from build123d import *

# Parameters (mm, degrees)
ESQUISSE2_W    = 4
ESQUISSE2_H    = 2
ESQUISSE2_W_2  = 2
ESQUISSE2_H_2  = 4
ENCOCHES_DEPTH = 24.34523506


with BuildPart() as part:
    # Esquisse1 → Base (revolve)
    with BuildSketch(Plane.XY, mode=Mode.PRIVATE) as base_sk:
        Polygon((7.633974596, 5), (14, 5), (14, 1.154700538), (12, 0), (7.633974596, 0), align=None)
    revolve(base_sk.sketch.rotate(Axis((0, 0, 0), (0, 1, 0)), 90), axis=Axis((0, 0, 0), (0, 1, 0)))

    # Esquisse2 → Encoches (cut, through all)
    with BuildSketch(Plane(origin=(0, 5, -4), x_dir=(1, 0, 0), z_dir=(0, -1, 0))):
        with Locations((0, -9)):
            Rectangle(ESQUISSE2_W, ESQUISSE2_H)
        with Locations((0, 17)):
            Rectangle(ESQUISSE2_W, ESQUISSE2_H)
        with Locations((13, 4)):
            Rectangle(ESQUISSE2_W_2, ESQUISSE2_H_2)
        with Locations((-13, 4)):
            Rectangle(ESQUISSE2_W_2, ESQUISSE2_H_2)
    extrude(amount=ENCOCHES_DEPTH, mode=Mode.SUBTRACT)


solid = part.part
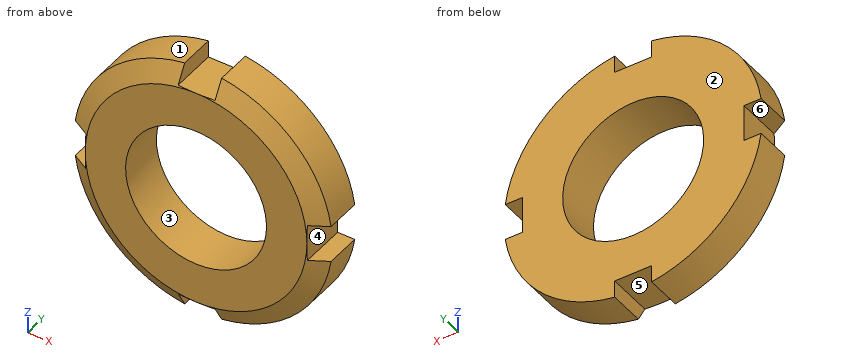
Build history of the part. All positions in model axes, mm. Face numbers are marked on the shaded views. A direction names the side the tool comes from. Coordinates: 2 decimals unless noted, no trailing zeros. Order: outer loops, then holes, each group sorted by start corner. A loop starts at its lowest first (then second) coordinate and runs counter-clockwise, first axis right, second up. Notation, with made-up numbers: (59, 86) - (97, 86) arc R16 ccw to (97, 101) - close; hole circle Ø2 at (9, -24.5). An arc over 180 degrees is marked (long way). Put each result on its own line as item: value.
1. Saw through at B-B (y = 0.8). Write the cut outline in (x, z), and give its area (3 significant figures).
Answer sheet:
outline: (-13.24, -2) arc R13.39 ccw to (-2, -13.24) - (-2, -12) - (2, -12) - (2, -13.24) arc R13.39 ccw to (13.24, -2) - (12, -2) - (12, 2) - (13.24, 2) arc R13.39 ccw to (2, 13.24) - (2, 12) - (-2, 12) - (-2, 13.24) arc R13.39 ccw to (-13.24, 2) - (-12, 2) - (-12, -2) - close; hole circle Ø15.27 at (0, 0)
area: 358 mm^2
2. Pull direction Z, two halves, no side cores. Call the marked faces 1, 2 and 3: pulls with the +Z half, pulls with the -Z half, needs draft (parallel to the pull), parting line crosses it, or undercut.
Answer sheet:
face 1: pulls with the +Z half
face 2: needs draft
face 3: undercut
3. Drop flat-ended pins along their axis: P1, Ø0.9, axis at x = 13, y = 3, coming from the -Z side; P2, Ø0.9, axis at x = 12.5, y = 2, coming from the +Z side; P3, Ø1.5, axis at x = -10.5, y = 3.5, coming from the -Z side. Give the stop position or say it passes through.
Answer sheet:
P1: stops at z = -6.2
P2: stops at z = 7.13
P3: stops at z = -10.05
4. Tool access for the marked faces 4, 5 and 6: list every direction of +Z, -Z, +X, -X, +Y, -Y with a clear straight run to the whole face (end or side of a thin tool).
Answer sheet:
face 4: +X, +Y, -Y
face 5: -Z, +Y, -Y
face 6: -X, +Y, -Y
5. Saw through at A-A (y = 2.25). Write the cut outline in (x, z).
Answer sheet:
outline: (-13.86, -2) arc R14 ccw to (-2, -13.86) - (-2, -12) - (2, -12) - (2, -13.86) arc R14 ccw to (13.86, -2) - (12, -2) - (12, 2) - (13.86, 2) arc R14 ccw to (2, 13.86) - (2, 12) - (-2, 12) - (-2, 13.86) arc R14 ccw to (-13.86, 2) - (-12, 2) - (-12, -2) - close; hole circle Ø15.27 at (0, 0)
6. Probe line 1 along X through (y, z) = (3.15, 0); line 2 along Z through (x, y) = (5.75, 3.6); line 3 along Z through (x, y) = (6.25, 3.8). List the from-to ranges inside material, lowest first. Write a range as [from, to].
Answer sheet:
line 1: x = [-12, -7.63], [7.63, 12]
line 2: z = [-12.76, -5.02], [5.02, 12.76]
line 3: z = [-12.53, -4.38], [4.38, 12.53]
